Part print with two shaded views. Sizes in mm from the minimum x, y, z corner. A direction names the side the tool comes from. Coordinates: 2 decimals unless noted, no trailing zeros. Write each loop counter-clockwise with the first axis right and the second up, starting at its lowest first coordinate (ties: lowest second). Pieces come first, ordered by that corner, then holes. Notation, with made-up numbers: (36, 39.5) - (95, 39.5) arc R24 ccw to (95, 70.5) - close; hole circle Ø10 at (-22, 23.5). An arc over 180 degrees is marked (long way). One line per question, with ' | ' between items. Start each with the question number.
1. Two-plate mould, pull along X, no slides. Class the marked faces 1, 2, 3 and 4: +X half, -X half, draft (parallel to the pull), parting line (faces both ways), or undercut.
2. Probe line 1 (Y direction, x = 4.75, z = 10); line 2 (X direction, y = 17.75, z = 16.5); line 3 (X direction, y = 9.25, z = 7.25). List the from-to ranges inside material, lowest first.
3. Band-saw the part on D-D, the plane y = 21. Write the cut outline in (x, z), then the cut area to 3 significant figures.
4. Band-saw the part on A-A, the plane y = 2.5. Write the cut outline in (x, z).
5. Which spindle directions (+Z, -Z, +X, -X, +Y, -Y) get a long thin tool onto all of the face, cutting with end or side? Do the marked faces 5, 6 and 7. Say none if no direction does.
6. Band-saw the part on C-C, the plane x = 9.5. Write the cut outline in (y, z), then the cut area to 4 significant figures.
7. Flat gauge pins, fed straight in: P1, Ø5, axis at x = 9.5, y = 21, coming from the +Z side; P2, Ø1.5, axis at y = 1.5, z = 9, coming from the +X side; P3, Ø8, axis at x = 9, y = 8, coming from the -Z side. Where does each tip first touch, or does it go through?
8. Band-saw the part on B-B, the plane z = 9.5. Write the cut outline in (x, y), then the cut area to 4 significant figures.
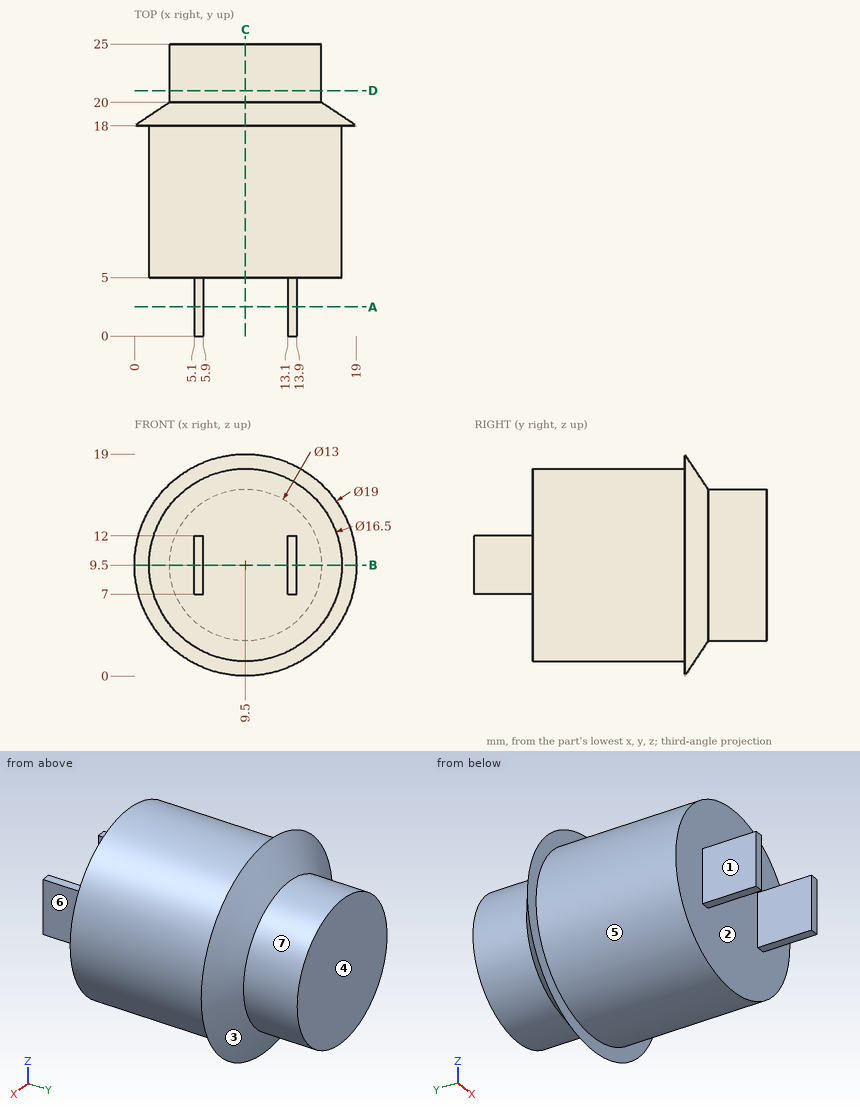
Filled in:
1) face 1: -X half | face 2: undercut | face 3: parting line | face 4: draft
2) line 1: y = 5 to 25 | line 2: x = 5.13 to 13.87 | line 3: x = 1.56 to 17.44
3) outline: circle Ø13 at (9.5, 9.5) | area: 133 mm²
4) outline: (5.1, 7) - (5.9, 7) - (5.9, 12) - (5.1, 12) - close; (13.1, 7) - (13.9, 7) - (13.9, 12) - (13.1, 12) - close
5) face 5: -Y | face 6: +Z, -Z, +X, -Y | face 7: +Y
6) outline: (5, 1.25) - (18, 1.25) - (18, 0) - (20, 3) - (25, 3) - (25, 16) - (20, 16) - (18, 19) - (18, 17.75) - (5, 17.75) - close | area: 311.5 mm²
7) P1: stops at z = 18.25 | P2: stops at x = 13.9 | P3: stops at z = 1.25
8) outline: (0, 18) - (1.25, 18) - (1.25, 5) - (5.1, 5) - (5.1, 0) - (5.9, 0) - (5.9, 5) - (13.1, 5) - (13.1, 0) - (13.9, 0) - (13.9, 5) - (17.75, 5) - (17.75, 18) - (19, 18) - (16, 20) - (16, 25) - (3, 25) - (3, 20) - close | area: 319.5 mm²
